from build123d import *

# Parameters (mm, degrees)
SKETCH_1_W          = 44
SKETCH_1_H          = 7.85
EXTRUDE_1_DEPTH     = 3
SKETCH_2_W          = 7.85
SKETCH_2_H          = 7
EXTRUDE_2_DEPTH     = 2
EXTRUDE_3_DEPTH     = 2
EXTRUDE_4_DEPTH     = 2
SKETCH_5_W          = 46
SKETCH_5_H          = 6.976539996
EXTRUDE_5_DEPTH     = 1
SKETCH_6_W          = 6
SKETCH_6_H          = 3
CUT_EXTRUDE_3_DEPTH = 3
SKETCH_8_W          = 3
SKETCH_8_H          = 6
CUT_EXTRUDE_4_DEPTH = 3


with BuildPart() as part:
    # 草图1 → 凸台-拉伸1 (new body)
    with BuildSketch(Plane(origin=(0, 0, 0), x_dir=(1, 0, 0), z_dir=(0, 1, 0))):
        with Locations((-13.612906347, -10.55497291)):
            Rectangle(SKETCH_1_W, SKETCH_1_H)
    extrude(amount=EXTRUDE_1_DEPTH)

    # 草图2 → 凸台-拉伸2 (add)
    with BuildSketch(Plane.ZY.offset(35.612906347)):
        with Locations((10.55497291, 3.5)):
            Rectangle(SKETCH_2_W, SKETCH_2_H)
    extrude(amount=EXTRUDE_2_DEPTH)

    # 草图3 → 凸台-拉伸3 (add)
    with BuildSketch(Plane.XY.offset(14.47997291)):
        Polygon((-35.612906347, 7), (-31.612906347, 3), (-31.612906347, 0), (-35.612906347, 0), (-37.612906347, 0), (-37.612906347, 7), align=None)
    extrude(amount=EXTRUDE_3_DEPTH)

    # 草图4 → 凸台-拉伸4 (add)
    with BuildSketch(Plane.XY.offset(14.47997291)):
        Polygon((8.387093653, 0), (8.387093653, 7), (4.387093653, 3), (4.387093653, 0), align=None)
    extrude(amount=EXTRUDE_4_DEPTH)

    # 草图5 → 凸台-拉伸5 (add)
    with BuildSketch(Plane(origin=(0, 0, 6.62997291), x_dir=(-1, 0, 0), z_dir=(0, 0, -1))):
        with Locations((14.612906347, 3.488269998)):
            Rectangle(SKETCH_5_W, SKETCH_5_H)
    extrude(amount=EXTRUDE_5_DEPTH)

    # 草图6 → 切除-拉伸3 (cut)
    with BuildSketch(Plane.XZ):
        with Locations((-14.612906347, 10.97997291)):
            Rectangle(SKETCH_6_W, SKETCH_6_H)
    extrude(amount=-CUT_EXTRUDE_3_DEPTH, mode=Mode.SUBTRACT)

    # 草图8 → 切除-拉伸4 (cut)
    with BuildSketch(Plane.XZ):
        with Locations((-14.612906347, 10.97997291)):
            Rectangle(SKETCH_8_W, SKETCH_8_H)
    extrude(amount=-CUT_EXTRUDE_4_DEPTH, mode=Mode.SUBTRACT)


solid = part.part
For this review, take the finished solid that the model builds, in its own axes (mm). A direction names the side the tool comes from. Round coordinates to 2 decimals unless told otherwise and drop trailing zeros. Order: outer loops, then holes, each group sorted by start corner. A loop starts at its lowest first (then second) coordinate and runs counter-clockwise, first axis right, second up. Notation, with made-up numbers: (34.5, -1) -> (79.5, -1) arc R5 ccw to (79.5, 8) -> close; hole circle Ø8 at (7, -24). An arc over 180 degrees is marked (long way). Write item = value, one per line. Start each with the question number.
1) Tool access review of faces 4 (the face through (-11.613, 1, 11)), 5 (the face through (-33.641, 5.028, 15.466)), 6 (the face through (-13, 1, 14.48)), 7 (the face through (-14, 3, 7)): name each direction out of +Z, -Z, +X, -X, +Y, -Y from which nothing blocks a thin tool from reaching the whole face with its end or side.
2) Take a section at A-A on z = 10.5. State the section outline as (x, y) points, plus the area to 3 significant figures.
3) Take a section at C-C on y = 1.75. State the section outline as (x, z) points, plus the area to 3 significant figures.
4) Take a section at B-B on y = 4.25. State the section outline as (x, z) points, plus the area to 3 significant figures.
5) Insertion check: pin 1 (1.5 mm diameter, centred on x = -32, z = 7, fed in from +Y); pin 2 (1.2 mm diameter, centred on x = -12.5, y = 1.5, fed in from +Z). Each pin has a flat end and moves straight along its axis. Give the tip position at first contact, or say it passes through.
6) To check wall thickness, follow line 1 (X direction, y = 2.75, z = 12.25); line 2 (Z direction, x = -33, y = 5.75); line 3 (X direction, y = 3.5, z = 11). State the ranges of each line that lie inside material, in increasing order. Write a range as from..to.
7) Take a section at D-D on x = -6. State the section outline as (y, z) points.
8) The part is to be moulded in two halves that separate along Z. For faces 1 (the face through (-35, 3, 16.48)), 2 (the face through (-16.113, 1, 9)), 3 (the face through (-37.613, 3, 11)), say which applies: +Z half, -Z half, draft (parallel to the pull), parting line (faces both ways), or undercut.
Verdict:
q1.face_4 = +Y, -Y
q1.face_5 = +Z, +Y
q1.face_6 = +Z, +Y, -Y
q1.face_7 = +X, +Y
q2.outline = (-37.61, 0) -> (-17.61, 0) -> (-17.61, 3) -> (-35.61, 3) -> (-35.61, 7) -> (-37.61, 7) -> close; (-11.61, 0) -> (8.39, 0) -> (8.39, 3) -> (-11.61, 3) -> close
q2.area = 128 mm2
q3.outline = (-37.61, 5.63) -> (8.39, 5.63) -> (8.39, 16.48) -> (4.39, 16.48) -> (4.39, 14.48) -> (-31.61, 14.48) -> (-31.61, 16.48) -> (-37.61, 16.48) -> close; hole (-17.61, 9.48) -> (-16.11, 9.48) -> (-16.11, 7.98) -> (-13.11, 7.98) -> (-13.11, 9.48) -> (-11.61, 9.48) -> (-11.61, 12.48) -> (-13.11, 12.48) -> (-13.11, 13.98) -> (-16.11, 13.98) -> (-16.11, 12.48) -> (-17.61, 12.48) -> close
q3.area = 400 mm2
q4.outline = (-37.61, 5.63) -> (8.39, 5.63) -> (8.39, 6.63) -> (-35.61, 6.63) -> (-35.61, 14.48) -> (-32.86, 14.48) -> (-32.86, 16.48) -> (-37.61, 16.48) -> close; (5.64, 14.48) -> (8.39, 14.48) -> (8.39, 16.48) -> (5.64, 16.48) -> close
q4.area = 76.7 mm2
q5.pin_1 = 6.98
q5.pin_2 = 14.48
q6.line_1 = -37.61..-17.61, -11.61..8.39
q6.line_2 = 5.63..6.63
q6.line_3 = -37.61..-35.61
q7.outline = (0, 5.63) -> (6.98, 5.63) -> (6.98, 6.63) -> (3, 6.63) -> (3, 14.48) -> (0, 14.48) -> close
q8.face_1 = +Z half
q8.face_2 = undercut
q8.face_3 = draft
